Part model, mm, in its own coordinate system. A direction names the side the tool comes from. Round coordinates to 2 decimals unless told otherwise and drop trailing zeros. Order: outer loops, then holes, each group sorted by start corner. A loop starts at its lowest first (then second) coordinate and runs counter-clockwise, first axis right, second up. Notation, with made-up numbers: (47, 43.5) -> (71, 43.5) arc R19 cw to (71, 77.5) -> close; hole circle Ø8 at (40.5, 2). An arc over 180 degrees is marked (long way). Use CSV: the item, a comma, the result in double quotes.
```python
from build123d import *

# Parameters (mm, degrees)
F0_R     = 10
F1_DEPTH = 25
F2_DEPTH = 50
F3_SIZE  = 2
F5_DEPTH = 25


with BuildPart() as f1:
    # F0 (on Front) → F1 (new body)
    with BuildSketch(Plane.XZ):
        with BuildLine():
            ThreePointArc((2.083333, -24.913043), (18.399502, -16.92508), (25, 0))
            ThreePointArc((25, 0), (18.399502, 16.92508), (2.083333, 24.913043))
            ThreePointArc((2.083333, 24.913043), (-25, 0), (2.083333, -24.913043))
        make_face()
        Circle(F0_R, mode=Mode.SUBTRACT)
        with BuildLine():
            ThreePointArc((2.083333, 24.913043), (18.399502, 16.92508), (25, 0))
            ThreePointArc((25, 0), (18.399502, -16.92508), (2.083333, -24.913043))
            Line((2.083333, -24.913043), (91.458333, -17.43913))
            ThreePointArc((91.458333, -17.43913), (72.5, 0), (91.458333, 17.43913))
            Line((91.458333, 17.43913), (2.083333, 24.913043))
        make_face()
        with BuildLine():
            ThreePointArc((107.5, 0), (102.879651, 11.847556), (91.458333, 17.43913))
            ThreePointArc((91.458333, 17.43913), (72.5, 0), (91.458333, -17.43913))
            ThreePointArc((91.458333, -17.43913), (102.879651, -11.847556), (107.5, 0))
        make_face()
        with Locations((90, 0)):
            Circle(F0_R, mode=Mode.SUBTRACT)
    extrude(amount=F1_DEPTH)

    # F0 (on Front) → F2 (join)
    with BuildSketch(Plane.XZ):
        with BuildLine():
            ThreePointArc((2.083333, -24.913043), (18.399502, -16.92508), (25, 0))
            ThreePointArc((25, 0), (18.399502, 16.92508), (2.083333, 24.913043))
            ThreePointArc((2.083333, 24.913043), (-25, 0), (2.083333, -24.913043))
        make_face()
        Circle(F0_R, mode=Mode.SUBTRACT)
    extrude(amount=F2_DEPTH)

    # F3
    f3_edges = [f1.edges().sort_by_distance(p)[0] for p in [
        (-2.083333, -50, 24.913043),
        (-10, -50, 0),
        (80, -25, 0),
    ]]
    chamfer(f3_edges, length=F3_SIZE)

    # F4 (on Top) → F5 (join)
    with BuildSketch(Plane.XY):
        Polygon((116.36319, -72.40244), (114.546522, 0), (94.42164, 29.210314), (-57.820518, 52.423224), (-47.972556, 0), (-15.099764, -72.40244), align=None)
    extrude(amount=F5_DEPTH)


solid = f1.part
```
(1) Cut at A-A, the plane x = 0. Give the cut face in (y, z).
Reply:
outline,"(-72.4, 0) -> (43.61, 0) -> (43.61, 25) -> (-72.4, 25) -> close; (-50, -23) -> (-48, -25) -> (0, -25) -> (0, -10) -> (-48, -10) -> (-50, -12) -> close"
(2) Cut at B-B, the plane y = -44. Give the cut face in (x, z), then the cut area to 3 significant figures.
Reply:
outline,"(-28, 0) -> (-25, 0) arc R25 ccw to (2.08, -24.91) arc R25 ccw to (25, 0) -> (115.65, 0) -> (115.65, 25) -> (-28, 25) -> close; hole (-10, 0) arc R10 ccw to (10, 0) -> close"
area,"4,420 mm2"
(3) Probe probe 1 along Y at (x, z) = (53, -12); probe 2 along Y at (x, z) = (-17.5, -9); probe 3 along Z at (x, y) = (72.5, -63.5). List the from-to ranges inside material, lowest first. Write a range as [from, to].
Reply:
probe 1,"[-25, 0]"
probe 2,"[-50, 0]"
probe 3,"[0, 25]"
(4) Drop flat-ended pins along their axis: P1, Ø2, axis at x = 75, y = 7.5, coming from the -Z side; P2, Ø7.5, axis at x = 62.5, z = -8.5, coming from the +Y side; P3, Ø4, axis at x = 68, y = -12, coming from the -Z side. Give the stop position or say it passes through.
Reply:
P1,"z = 0"
P2,"y = 0"
P3,"z = -19.57"
(5) Pull direction Z, two halves, no side cores. Call faces 6 (the face through (46.15, -12.32, -21.23)), 7 (the face through (50, -72.402, 12)), 8 (the face through (90, -11, -10)): released by +Z, released by -Z, zero draft, split by the parting line, or undercut.
Reply:
face 6,"released by -Z"
face 7,"zero draft"
face 8,"undercut"
(6) Cut at C-C, the plane z = 8. Give the cut face in (x, y).
Reply:
outline,"(-57.82, 52.42) -> (-47.97, 0) -> (-15.1, -72.4) -> (116.36, -72.4) -> (114.55, 0) -> (94.42, 29.21) -> close"
(7) Cut at D-D, the plane x = 70. Give the cut face in (y, z).
Reply:
outline,"(-72.4, 0) -> (-25, 0) -> (-25, -19.23) -> (0, -19.23) -> (0, 0) -> (32.93, 0) -> (32.93, 25) -> (-72.4, 25) -> close"
(8) Which spindle directions (+Z, -Z, +X, -X, +Y, -Y) get a long thin tool onto all of the face, cutting with end or side? Do faces 1 (the face through (89.777, -23.125, -10.123)), 2 (the face through (0, -50, -14)), 3 (the face through (54, -25, -12)), 4 (the face through (0, -24, -10)), 5 (the face through (40, 0, -12)). Say none if no direction does.
Reply:
face 1,"-Y"
face 2,"-Z, +X, -X, -Y"
face 3,"-Z, +X, -Y"
face 4,"+Y, -Y"
face 5,"-Z, +X, -X, +Y"
